Source: CAD feature listing. Evaluate the final solid. Frame: model axes, mm. A direction names the side the tool comes from. Round coordinates to 2 decimals unless told otherwise and drop trailing zeros. Order: outer loops, then holes, each group sorted by start corner. A loop starts at its lowest first (then second) coordinate and runs counter-clockwise, first axis right, second up.
Autodesk Inventor part; units mm, degrees
ref_plane "YZ Plane" through (0, 0, 0) normal (1, 0, 0) x (0, 1, 0)
ref_plane "XZ Plane" through (0, 0, 0) normal (0, 1, 0) x (-1, 0, 0)
ref_plane "XY Plane" through (0, 0, 0) normal (0, 0, 1) x (1, 0, 0)
sketch "Esquisse1" plane through (0, 0, 0) normal (0, 1, 0) x (-1, 0, 0)
  circle A0 centre (0, 0) radius 11
  dimension "d1" = 22
extrude "Extrusion1" add sketch "Esquisse1" along normal blind 5
sketch "Esquisse2" plane through (0, 5, 0) normal (0, 1, 0) x (1, 0, 0)
  arc A0 (-10, 0) -> (10, 0) centre (0, 0) ccw
  line L0 (-10, 0) -> (10, 0)
  dimension "d4" = 20
revolve "Révolution1" add sketch "Esquisse2" angle 180 about axis through (-10, 5, 0) along (-1, 0, 0)
ref_plane "Plan de construction1" through (16.1473, 5, 0) normal (1, 0, 0) x (0, 0, -1)
sketch "Esquisse6" plane through (16.1473, 5, 0) normal (1, 0, 0) x (0, 0, -1)
  circle A0 centre (0, -2.5) radius 1.35
  point P0 (0, -5)
  point P1 (0, -1.15)
  dimension "d11" = 2.7
extrude "Extrusion4" add sketch "Esquisse6" against normal blind 5.25
sketch "Esquisse7" plane through (0, 0, 0) normal (0, -1, 0) x (1, 0, 0)
  circle A0 centre (0, 9.5) radius 1
  circle A1 centre (0, -9.5) radius 1
  circle A2 centre (-9.5, 0) radius 1
  point P0 (0, 0)
  dimension "d15" = 2
  dimension "d16" = 2
  dimension "d17" = 2
extrude "Extrusion5" cut sketch "Esquisse7" against normal blind 4
properties part number "Capteur optoforce"
1. Section B-B on x = 0. Return loops of the section in (y, z), plus the area to 3 significant figures.
2. Line query: line 1 along Z through (x, y) = (0, 2.75); line 2 along Y through (x, z) = (5.25, -8.75); line 3 along Z through (x, y) = (-9.5, 3.1). Output: solid intervals per line, ascending.
3. Pull-direction query (X, two-part tool) for faces 4 (the face through (-2, 5, -10)), 5 (the face through (0, 4, -9)), 6 (the face through (-10.161, 2.465, 4.213)); classes: released by +X, released by -X, zero draft, split by the parting line, or undercut.
4. Access query for faces 1 (the face through (13.57, 1.18, 0.29)), 2 (the face through (0, 4, 10)), 3 (the face through (0, 0, 0)). Directions: +Z, -Z, +X, -X, +Y, -Y. A direction counts if a zero-diameter tool reaches every point of the face in a straight line with its end or side. Return the directions, or none.
5. Section D-D on z = 9. Return loops of the section in (x, y), plus the area to 3 significant figures.
6. First-contact query: pin 1 (0.6 mm diameter, centred on x = -9.5, z = 0, fed in from -Y); pin 2 (6 mm diameter, centred on x = -7.5, z = 3, fed in from +Y); pin 3 (6 mm diameter, centred on x = 1.5, z = 1.5, fed in from +Y). Flat tips, straight axial feed; report the tip coordinate or a pass-through.
7. Section A-A on z = 0. Return loops of the section in (x, y).
8. Section C-C on y = 4.5. Return loops of the section in (x, z), plus the area to 3 significant figures.
Result:
1. outline: (0, -11) - (5, -11) - (5, -10) arc R10 ccw to (5, 10) - (5, 11) - (0, 11) - (0, 10.5) - (4, 10.5) - (4, 8.5) - (0, 8.5) - (0, -8.5) - (4, -8.5) - (4, -10.5) - (0, -10.5) - close
1. area: 251 mm2
2. line 1: z = -11 to -10.5, -8.5 to 8.5, 10.5 to 11
2. line 2: y = 0 to 5
2. line 3: z = -5.55 to -1, 1 to 5.55
3. face 4: zero draft
3. face 5: undercut
3. face 6: split by the parting line
4. face 1: +X
4. face 2: -Y
4. face 3: +Z, -Z, +X, -X, -Y
5. outline: (-6.32, 0) - (-0.87, 0) - (-0.87, 4) - (0.87, 4) - (0.87, 0) - (6.32, 0) - (6.32, 5) - (4.36, 5) arc R4.36 ccw to (-4.36, 5) - (-6.32, 5) - close
5. area: 86.2 mm2
6. pin 1: stops at y = 4
6. pin 2: stops at y = 13.61
6. pin 3: stops at y = 15
7. outline: (-11, 0) - (-10.5, 0) - (-10.5, 4) - (-8.5, 4) - (-8.5, 0) - (11, 0) - (11, 1.15) - (16.15, 1.15) - (16.15, 3.85) - (11, 3.85) - (11, 5) - (10, 5) arc R10 ccw to (-10, 5) - (-11, 5) - close
8. outline: circle Ø22 at (0, 0)
8. area: 380 mm2
